```python
from build123d import *

# Parameters (mm, degrees)
SKETCH1_W           = 120
SKETCH1_H           = 70
BOSS_EXTRUDE1_DEPTH = 5
FILLET1_R           = 6
BOSS_EXTRUDE2_DEPTH = 3
SKETCH3_R           = 5.5
CUT_EXTRUDE1_DEPTH  = 2
SKETCH4_R           = 3.2
CUT_EXTRUDE2_DEPTH  = 2
SKETCH5_R           = 1.7
CUT_EXTRUDE3_DEPTH  = 70.720872054
CUT_EXTRUDE4_DEPTH  = 1
SKETCH7_W           = 30
SKETCH7_H           = 30
CUT_EXTRUDE5_DEPTH  = 0.8


with BuildPart() as part:
    # Sketch1 → Boss-Extrude1 (new body)
    with BuildSketch(Plane.XY):
        Rectangle(SKETCH1_W, SKETCH1_H)
    extrude(amount=BOSS_EXTRUDE1_DEPTH)

    # Fillet1
    fillet1_edges = [part.edges().sort_by_distance(p)[0] for p in [
        (-60, 35, 2.5),
        (60, 35, 2.5),
        (60, -35, 2.5),
        (-60, -35, 2.5),
    ]]
    fillet(fillet1_edges, radius=FILLET1_R)

    # Sketch2 → Boss-Extrude2 (add)
    with BuildSketch(Plane(origin=(0, 0, 0), x_dir=(-1, 0, 0), z_dir=(0, 0, -1))):
        with BuildLine():
            Line((-53.75, 31.75), (53.75, 31.75))
            ThreePointArc((53.75, 31.75), (55.871320344, 30.871320344), (56.75, 28.75))
            Line((56.75, 28.75), (56.75, -28.75))
            ThreePointArc((56.75, -28.75), (55.871320344, -30.871320344), (53.75, -31.75))
            Line((53.75, -31.75), (-53.75, -31.75))
            ThreePointArc((-53.75, -31.75), (-55.871320344, -30.871320344), (-56.75, -28.75))
            Line((-56.75, -28.75), (-56.75, 28.75))
            ThreePointArc((-56.75, 28.75), (-55.871320344, 30.871320344), (-53.75, 31.75))
        make_face()
        with BuildLine():
            Line((-51.75, 29.75), (51.75, 29.75))
            ThreePointArc((51.75, 29.75), (53.871320344, 28.871320344), (54.75, 26.75))
            Line((54.75, 26.75), (54.75, -26.75))
            ThreePointArc((54.75, -26.75), (53.871320344, -28.871320344), (51.75, -29.75))
            Line((51.75, -29.75), (-51.75, -29.75))
            ThreePointArc((-51.75, -29.75), (-53.871320344, -28.871320344), (-54.75, -26.75))
            Line((-54.75, -26.75), (-54.75, 26.75))
            ThreePointArc((-54.75, 26.75), (-53.871320344, 28.871320344), (-51.75, 29.75))
        make_face(mode=Mode.SUBTRACT)
    extrude(amount=BOSS_EXTRUDE2_DEPTH)

    # Sketch3 → Cut-Extrude1 (cut)
    with BuildSketch(Plane(origin=(0, 0, -3), x_dir=(-1, 0, 0), z_dir=(0, 0, -1))):
        with Locations((-52, 27)):
            Circle(SKETCH3_R)
        with Locations((-52, -27)):
            Circle(SKETCH3_R)
        with Locations((52, -27)):
            Circle(SKETCH3_R)
        with Locations((52, 27)):
            Circle(SKETCH3_R)
    extrude(amount=-CUT_EXTRUDE1_DEPTH, mode=Mode.SUBTRACT)

    # Sketch4 → Cut-Extrude2 (cut)
    with BuildSketch(Plane.XY.offset(5)):
        with Locations((52, 27)):
            Circle(SKETCH4_R)
        with Locations(Location((52, -27, 0), (0, 0, 180))):
            Circle(SKETCH4_R)
        with Locations((-52, -27)):
            Circle(SKETCH4_R)
        with Locations(Location((-52, 27, 0), (0, 0, 180))):
            Circle(SKETCH4_R)
    extrude(amount=-CUT_EXTRUDE2_DEPTH, mode=Mode.SUBTRACT)

    # Sketch5 → Cut-Extrude3 (cut, through all)
    with BuildSketch(Plane.XY.offset(3)):
        with Locations((52, 27)):
            Circle(SKETCH5_R)
        with Locations((52, -27)):
            Circle(SKETCH5_R)
        with Locations((-52, -27)):
            Circle(SKETCH5_R)
        with Locations((-52, 27)):
            Circle(SKETCH5_R)
    extrude(amount=-CUT_EXTRUDE3_DEPTH, mode=Mode.SUBTRACT)

    # Sketch6 → Cut-Extrude4 (cut)
    with BuildSketch(Plane(origin=(0, 0, 0), x_dir=(-1, 0, 0), z_dir=(0, 0, -1))):
        with BuildLine():
            Line((-54, 34.1), (54, 34.1))
            ThreePointArc((54, 34.1), (57.606244584, 32.606244584), (59.1, 29))
            Line((59.1, 29), (59.1, -29))
            ThreePointArc((59.1, -29), (57.606244584, -32.606244584), (54, -34.1))
            Line((54, -34.1), (-54, -34.1))
            ThreePointArc((-54, -34.1), (-57.606244584, -32.606244584), (-59.1, -29))
            Line((-59.1, -29), (-59.1, 29))
            ThreePointArc((-59.1, 29), (-57.606244584, 32.606244584), (-54, 34.1))
        make_face()
        with BuildLine():
            Line((-54, 32.9), (54, 32.9))
            ThreePointArc((54, 32.9), (56.757716447, 31.757716447), (57.9, 29))
            Line((57.9, 29), (57.9, -29))
            ThreePointArc((57.9, -29), (56.757716447, -31.757716447), (54, -32.9))
            Line((54, -32.9), (-54, -32.9))
            ThreePointArc((-54, -32.9), (-56.757716447, -31.757716447), (-57.9, -29))
            Line((-57.9, -29), (-57.9, 29))
            ThreePointArc((-57.9, 29), (-56.757716447, 31.757716447), (-54, 32.9))
        make_face(mode=Mode.SUBTRACT)
    extrude(amount=-CUT_EXTRUDE4_DEPTH, mode=Mode.SUBTRACT)

    # Sketch7 → Cut-Extrude5 (cut)
    with BuildSketch(Plane.XY.offset(5)):
        with Locations((-33, 2)):
            Rectangle(SKETCH7_W, SKETCH7_H)
    extrude(amount=-CUT_EXTRUDE5_DEPTH, mode=Mode.SUBTRACT)


solid = part.part
```
Model file for the job. Use its own axes, mm. A direction names the side the tool comes from. Coordinates: 2 decimals unless noted, no trailing zeros. Loops run counter-clockwise (first coordinate to the right, second up) from the corner with the lowest first, then second, coordinate; pieces in that order, holes last. Notation, with made-up numbers: (-22, 17.25) - (8, 17.25) arc R30 ccw to (8, 51.25) - close; hole circle Ø6 at (32, 26.25). An arc over 180 degrees is marked (long way). Answer as a JSON object with one key per item and string values. Group by question number.
(1) Probe line 1 along Y through (x, z) = (52, 3.5); line 2 along Y through (x, z) = (-52, 1.8); line 3 along X through (y, z) = (-6.5, 4.5). List the from-to ranges inside material, lowest first.
(2) Two-plate mould, pull along X, no slides. Class faces 4 (the face through (56.75, 0, -1)), 5 (the face through (-56.75, 0, -1)), 6 (the face through (50.6, -25.6, 3)): released by +X, released by -X, zero draft, split by the parting line, or undercut.
(3) Flat gauge pins, fed straight in: pin 1 (3 mm diameter, centred on x = -33.5, y = 9.5, fed in from +Z); pin 2 (7 mm diameter, centred on x = -52.5, y = 27.5, fed in from +Z); pin 3 (5 mm diameter, centred on x = 49.5, y = 26, fed in from -Z); pin 4 (1.5 mm diameter, centred on y = -6, z = -1, fed in from -X). Where does each tip first touch, or does it go through?
(4) Cut at B-B (x = 35). Give the cut face in (y, z).
(5) Cut at C-C (y = -20). Give the cut face in (x, z), then the cut area to 3 significant figures.
(6) Cut at A-A (y = 2.5). Give the cut face in (x, z).
(7) Tool access for faces 1 (the face through (-52.417, -23.827, 4.014)), 2 (the face through (55.85, -30.89, -0.49)), 3 (the face through (-55.89, -30.85, -0.49)): list every direction of +Z, -Z, +X, -X, +Y, -Y with a clear straight run to the whole face (end or side of a thin tool).
Geometry says:
{
 "1": {"line 1": "y = -35 to -30.2, -23.8 to 23.8, 30.2 to 35", "line 2": "y = -35 to -28.7, -25.3 to 25.3, 28.7 to 35", "line 3": "x = -60 to -48, -18 to 60"},
 "2": {"face 4": "released by +X", "face 5": "released by -X", "face 6": "undercut"},
 "3": {"pin 1": "stops at z = 4.2", "pin 2": "stops at z = 5", "pin 3": "stops at z = 0", "pin 4": "stops at x = -56.75"},
 "4": {"outline": "(-35, 0) - (-34.1, 0) - (-34.1, 1) - (-32.9, 1) - (-32.9, 0) - (-31.75, 0) - (-31.75, -3) - (-29.75, -3) - (-29.75, 0) - (29.75, 0) - (29.75, -3) - (31.75, -3) - (31.75, 0) - (32.9, 0) - (32.9, 1) - (34.1, 1) - (34.1, 0) - (35, 0) - (35, 5) - (-35, 5) - close"},
 "5": {"outline": "(-60, 0) - (-59.1, 0) - (-59.1, 1) - (-57.9, 1) - (-57.9, 0) - (-56.75, 0) - (-56.75, -3) - (-54.75, -3) - (-54.75, 0) - (54.75, 0) - (54.75, -3) - (56.75, -3) - (56.75, 0) - (57.9, 0) - (57.9, 1) - (59.1, 1) - (59.1, 0) - (60, 0) - (60, 5) - (-60, 5) - close", "area": "610 mm^2"},
 "6": {"outline": "(-60, 0) - (-59.1, 0) - (-59.1, 1) - (-57.9, 1) - (-57.9, 0) - (-56.75, 0) - (-56.75, -3) - (-54.75, -3) - (-54.75, 0) - (54.75, 0) - (54.75, -3) - (56.75, -3) - (56.75, 0) - (57.9, 0) - (57.9, 1) - (59.1, 1) - (59.1, 0) - (60, 0) - (60, 5) - (-18, 5) - (-18, 4.2) - (-48, 4.2) - (-48, 5) - (-60, 5) - close"},
 "7": {"face 1": "+Z", "face 2": "-Z, +X, -Y", "face 3": "-Z, -X, -Y"}
}
